Part model, mm, in its own coordinate system. A direction names the side the tool comes from. Round coordinates to 2 decimals unless told otherwise and drop trailing zeros. Loops run counter-clockwise (first coordinate to the right, second up) from the corner with the lowest first, then second, coordinate; pieces in that order, holes last. Notation, with made-up numbers: (79, 11) -> (122, 11) arc R21 ccw to (122, 40) -> close; hole circle Ø4 at (-30, 4.5). An arc over 180 degrees is marked (long way). Use a Markdown table: item, result. Add a question column.
Item 1: Flat gauge pins, fed straight in: pin 1 (4 mm diameter, centred on x = -7.5, z = 0, fed in from +Y); pin 2 (1 mm diameter, centred on x = -1, z = -0.5, fed in from +Y). Where does each tip first touch, or does it go through?
Item 2: Cut at A-A, the plane y = 4.65. List the corners of the cut face in (x, z).
Item 3: Probe line 1 (X direction, y = 3.9, z = 0); line 2 (X direction, y = 3.6, z = -1.5); line 3 (Y direction, x = 3, z = -2.5). List the from-to ranges inside material, lowest first. Write a range as [from, to].
Item 4: Which spindle directions (+Z, -Z, +X, -X, +Y, -Y) get a long thin tool onto all of the face, cutting with end or side? Do faces 5 (the face through (12.559, 2.535, -3.508)), 6 (the face through (5.06, 3.87, -0.54)). Say none if no direction does.
Item 5: Two-plate mould, pull along Z, no slides. Class faces 1 (the face through (11, 5, 0)), 2 (the face through (0, 2, -4.5)), 3 (the face through (12.508, 2.535, 3.559)), 4 (the face through (8, 2.7, 0)): pulls with the +Z half, pulls with the -Z half, needs draft (parallel to the pull), parting line crosses it, or undercut.
Item 6: Cut at D-D, the plane x = 0. List the corners of the cut face in (y, z).
Item 7: Cut at C-C, the plane z = 3. List the corners of the cut face in (x, y).
Item 8: Cut at B-B, the plane y = 0.95. List the corners of the cut face in (x, z), plus the area to 3 significant figures.
```python
from build123d import *

# Parameters (mm, degrees)
SKETCH1_W           = 27
SKETCH1_H           = 9
BOSS_EXTRUDE1_DEPTH = 5
FILLET1_R           = 3.3
SKETCH2_R           = 2.5
CUT_EXTRUDE1_DEPTH  = 2.3
CUT_EXTRUDE4_DEPTH  = 2.5


with BuildPart() as part:
    # Sketch1 → Boss-Extrude1 (new body)
    with BuildSketch(Plane(origin=(0, 0, 0), x_dir=(1, 0, 0), z_dir=(0, 1, 0))):
        Rectangle(SKETCH1_W, SKETCH1_H)
    extrude(amount=BOSS_EXTRUDE1_DEPTH)

    # Fillet1
    fillet1_edges = [part.edges().sort_by_distance(p)[0] for p in [
        (13.5, 2.5, 4.5),
        (-13.5, 2.5, 4.5),
        (-13.5, 2.5, -4.5),
        (13.5, 2.5, -4.5),
    ]]
    fillet(fillet1_edges, radius=FILLET1_R)

    # Sketch2 → Cut-Extrude1 (cut)
    with BuildSketch(Plane(origin=(0, 5, 0), x_dir=(1, 0, 0), z_dir=(0, 1, 0))):
        with Locations(Location((-7.5, 0, 0), (0, 0, 270))):
            Circle(SKETCH2_R)
        with Locations(Location((7.5, 0, 0), (0, 0, 270))):
            Circle(SKETCH2_R)
    extrude(amount=-CUT_EXTRUDE1_DEPTH, mode=Mode.SUBTRACT)

    # Sketch4 → Cut-Extrude4 (cut)
    with BuildSketch(Plane(origin=(0, 5, 0), x_dir=(1, 0, 0), z_dir=(0, 1, 0))):
        with BuildLine():
            ThreePointArc((-3, 0), (-4.318019485, -3.181980515), (-7.5, -4.5))
            Line((-7.5, -4.5), (7.499999999, -4.5))
            ThreePointArc((7.499999999, -4.5), (3, 0), (7.5, 4.5))
            Line((7.5, 4.5), (-7.5, 4.5))
            ThreePointArc((-7.5, 4.5), (-4.318019485, 3.181980515), (-3, 0))
        make_face()
    extrude(amount=-CUT_EXTRUDE4_DEPTH, mode=Mode.SUBTRACT)


solid = part.part
```
A:
| question | item | result |
|---|---|---|
| 1 | pin 1 | stops at y = 2.7 |
| 1 | pin 2 | stops at y = 2.5 |
| 2 | outline | (-13.5, -1.2) arc R3.3 ccw to (-10.2, -4.5) -> (-7.5, -4.5) arc R4.5 ccw to (-7.5, 4.5) -> (-10.2, 4.5) arc R3.3 ccw to (-13.5, 1.2) -> close; (7.5, -4.5) -> (10.2, -4.5) arc R3.3 ccw to (13.5, -1.2) -> (13.5, 1.2) arc R3.3 ccw to (10.2, 4.5) -> (7.5, 4.5) arc R4.5 ccw to start; hole circle Ø5 at (-7.5, 0); hole circle Ø5 at (7.5, 0) |
| 3 | line 1 | x = [-13.5, -10], [-5, -3], [3, 5], [10, 13.5] |
| 3 | line 2 | x = [-13.49, -9.5], [-5.5, -3.26], [3.26, 5.5], [9.5, 13.49] |
| 3 | line 3 | y = [0, 2.5] |
| 4 | face 5 | -Z, +X, +Y, -Y |
| 4 | face 6 | +Y |
| 5 | face 1 | needs draft |
| 5 | face 2 | pulls with the -Z half |
| 5 | face 3 | pulls with the +Z half |
| 5 | face 4 | undercut |
| 6 | outline | (0, -4.5) -> (2.5, -4.5) -> (2.5, 4.5) -> (0, 4.5) -> close |
| 7 | outline | (-12.97, 0) -> (12.97, 0) -> (12.97, 5) -> (4.15, 5) -> (4.15, 2.5) -> (-4.15, 2.5) -> (-4.15, 5) -> (-12.97, 5) -> close |
| 8 | outline | (-13.5, -1.2) arc R3.3 ccw to (-10.2, -4.5) -> (10.2, -4.5) arc R3.3 ccw to (13.5, -1.2) -> (13.5, 1.2) arc R3.3 ccw to (10.2, 4.5) -> (-10.2, 4.5) arc R3.3 ccw to (-13.5, 1.2) -> close |
| 8 | area | 234 mm^2 |
